The drawing under review shows one solid part. Ordinate dimensions are in mm from its lowest x, y, z. A direction names the side the tool comes from. Coordinates: 2 decimals unless noted, no trailing zeros. Write each loop counter-clockwise with the first axis right and the second up, starting at its lowest first coordinate (ties: lowest second). Pieces come first, ordered by that corner, then holes.
Q1. Add section C-C, the plane x = 31.5. Give the boundary of the cut face in (y, z), plus the area to 3 significant figures.
Q2. The part is to be moulded in two halves that separate along X. For the marked faces 1, 2 and 3, say which applies: +X half, -X half, draft (parallel to the pull), parting line (faces both ways), or undercut.
Q3. Add section D-D, the plane z = 63. Give the boundary of the cut face in (x, y).
Q4. Machinability: for the marked faces 4 and 5, which of the approach directions +Z, -Z, +X, -X, +Y, -Y give a long, thin tool a straight path to every point of the face, cutting with its end or side? Answer none if there is none.
Q5. Add section A-A, the plane z = 7. Give the boundary of the cut face in (x, y), plus the area to 3 significant figures.
Q6. Clearance check with flat-ended pins moving along their axes: pin 1 Ø4 at (x, y) = (36.5, 35.5) entering from -Z; pin 2 Ø2.5 at (x, z) = (2.5, 2.5) entering from -Y. State where each tip first meets the part, or that it passes through.
Q7. To check wall thickness, follow probe 1 along Z at (x, y) = (2.5, 2.6); probe 2 along X at (y, z) = (3, 51); probe 3 along Z at (x, y) = (57, 37.5). State the ranges of each line that lie inside material, in increasing order.
Q8. Add section B-B, the plane y = 47.5. Give the boundary of the cut face in (x, z).
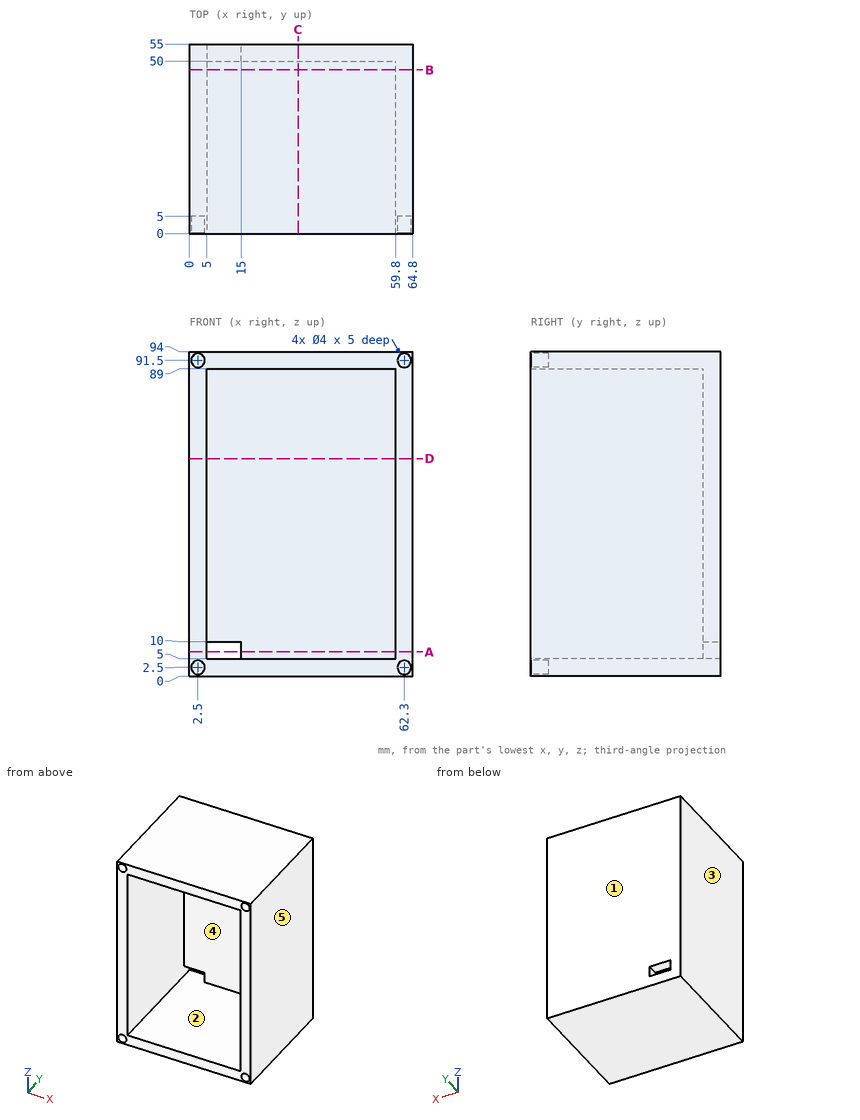
Here are the results:
1. outline: (0, 0) - (55, 0) - (55, 94) - (0, 94) - (0, 89) - (50, 89) - (50, 5) - (0, 5) - close
1. area: 970 mm2
2. face 1: draft
2. face 2: undercut
2. face 3: -X half
3. outline: (0, 0) - (5, 0) - (5, 50) - (59.8, 50) - (59.8, 0) - (64.8, 0) - (64.8, 55) - (0, 55) - close
4. face 4: -Y
4. face 5: +Z, -Z, +X, +Y, -Y
5. outline: (0, 0) - (5, 0) - (5, 55) - (0, 55) - close; (15, 50) - (59.8, 50) - (59.8, 0) - (64.8, 0) - (64.8, 55) - (15, 55) - close
5. area: 774 mm2
6. pin 1: stops at z = 0
6. pin 2: stops at y = 5
7. probe 1: z = 0 to 0.5, 4.5 to 89.5, 93.5 to 94
7. probe 2: x = 0 to 5, 59.8 to 64.8
7. probe 3: z = 0 to 5, 89 to 94
8. outline: (0, 0) - (64.8, 0) - (64.8, 94) - (0, 94) - close; hole (5, 5) - (59.8, 5) - (59.8, 89) - (5, 89) - close
